from build123d import *

# Parameters (mm, degrees)
SKETCH2_R           = 6
BOSS_EXTRUDE1_DEPTH = 20
SKETCH3_R           = 10
BOSS_EXTRUDE2_DEPTH = 2
CHAMFER1_SIZE       = 0.6
CHAMFER2_SIZE       = 0.3


with BuildPart() as part:
    # Sketch2 → Boss-Extrude1 (new body)
    with BuildSketch(Plane.XY):
        Circle(SKETCH2_R)
    extrude(amount=BOSS_EXTRUDE1_DEPTH)

    # Sketch3 → Boss-Extrude2 (add)
    with BuildSketch(Plane.XY.offset(20)):
        Circle(SKETCH3_R)
    extrude(amount=BOSS_EXTRUDE2_DEPTH)

    # Chamfer1
    chamfer1_edges = [part.edges().sort_by_distance(p)[0] for p in [
        (-6, 0, 0),
    ]]
    chamfer(chamfer1_edges, length=CHAMFER1_SIZE)

    # Chamfer2
    chamfer2_edges = [part.edges().sort_by_distance(p)[0] for p in [
        (-10, 0, 20),
        (-10, 0, 22),
    ]]
    chamfer(chamfer2_edges, length=CHAMFER2_SIZE)


solid = part.part
Can you work these out from the model? Positions are in its coordinate system, mm. A direction names the side the tool comes from. Give positions to 0.01 mm unless a question says otherwise; leave off trailing zeros. Order: outer loops, then holes, each group sorted by start corner. A loop starts at its lowest first (then second) coordinate and runs counter-clockwise, first axis right, second up. Notation, with made-up numbers: M 84.5,-19.75 L 134.5,-19.75 A12 cw 134.5,-11.75 Z; hole C 38,-19.5 d2. An arc over 180 degrees is marked long. Use a Markdown table: item, result. Add a question column.
Item 1: Will these pins go through, and if not, where does the flat tip stop? pin 1 (2 mm diameter, centred on y = -8, z = 2.5, fed in from +X); pin 2 (1 mm diameter, centred on y = 1, z = 4.5, fed in from +X); pin 3 (5 mm diameter, centred on x = -5.5, z = 3.5, fed in from -Y); pin 4 (2 mm diameter, centred on y = 2, z = 18.5, fed in from +X).
Item 2: Suppose I cut it at A-A (y = 0). List the corners of the cut face in (x, z) for me.
Item 3: For faces 1 (the cylindrical face through (-2.17, -9.76, 20.99)), 2 (the cylindrical face through (-6, 0, 10)), which set-ups out of +Z, -Z, +X, -X, +Y, -Y let a thin tool reach every point of the face, with its end or its side?
Item 4: Suppose I cut it at C-C (z = 20.75). List the corners of the cut face in (x, y) for me, then the cut area to 3 significant figures.
Item 5: If I drill on L1, parallel to Z at x = 0.75, y = -6; L2, parallel to X at y = -0.25, z = 6; L3, parallel to X at y = 4.5, z = 2.5, over which ranges is the centre line in solid material (lowest first)? Write a range as [from, to].
Item 6: Suppose I cut it at D-D (z = 14.75). List the corners of the cut face in (x, y) for me.
Answer sheet:
| question | item | result |
|---|---|---|
| 1 | pin 1 | passes through |
| 1 | pin 2 | stops at x = 5.98 |
| 1 | pin 3 | stops at y = -5.2 |
| 1 | pin 4 | stops at x = 5.92 |
| 2 | outline | M -10,20.3 L -9.7,20 L -6,20 L -6,0.6 L -5.4,0 L 5.4,0 L 6,0.6 L 6,20 L 9.7,20 L 10,20.3 L 10,21.7 L 9.7,22 L -9.7,22 L -10,21.7 Z |
| 3 | face 1 | +Z, -Z |
| 3 | face 2 | -Z |
| 4 | outline | C 0,0 d20 |
| 4 | area | 314 mm² |
| 5 | L1 | z = [20, 22] |
| 5 | L2 | x = [-5.99, 5.99] |
| 5 | L3 | x = [-3.97, 3.97] |
| 6 | outline | C 0,0 d12 |
